Autodesk Inventor part; units mm, degrees
ref_plane "Počáteční rovina" through (0, 0, 0) normal (0, 0, 1) x (1, 0, 0)
ref_plane "Koncová rovina" through (0, 0, 1075) normal (0, 0, 1) x (1, 0, 0)
ref_plane "YZ Plane" through (0, 0, 0) normal (1, 0, 0) x (0, 1, 0)
ref_plane "Počáteční rovina" through (0, 0, 0) normal (0, 0, 1) x (1, 0, 0)
ref_plane "Koncová rovina" through (0, 0, 1075) normal (0, 0, 1) x (1, 0, 0)
sketch "Náčrt1" plane through (0, 0, 0) normal (0, 0, 1) x (1, 0, 0)
  line L0 (-11.5, 17.5) -> (11.5, 17.5)
  line L1 (17.5, 11.5) -> (17.5, -11.5)
  line L2 (11.5, -17.5) -> (-11.5, -17.5)
  line L3 (-17.5, -11.5) -> (-17.5, 11.5)
  arc A0 (-11.5, 17.5) -> (-17.5, 11.5) centre (-11.5, 11.5) ccw
  arc A1 (17.5, 11.5) -> (11.5, 17.5) centre (11.5, 11.5) ccw
  arc A2 (11.5, -17.5) -> (17.5, -11.5) centre (11.5, -11.5) ccw
  arc A3 (-17.5, -11.5) -> (-11.5, -17.5) centre (-11.5, -11.5) ccw
  line L4 (-21.8698, 0) -> (21.8698, 0) construction
  line L5 (0, -21.8698) -> (0, 21.8698) construction
  arc A4 (-11.5, 14.5) -> (-14.5, 11.5) centre (-11.5, 11.5) ccw
  line L6 (-11.5, 14.5) -> (11.5, 14.5)
  arc A5 (14.5, 11.5) -> (11.5, 14.5) centre (11.5, 11.5) ccw
  line L7 (14.5, 11.5) -> (14.5, -11.5)
  arc A6 (11.5, -14.5) -> (14.5, -11.5) centre (11.5, -11.5) ccw
  line L8 (11.5, -14.5) -> (-11.5, -14.5)
  arc A7 (-14.5, -11.5) -> (-11.5, -14.5) centre (-11.5, -11.5) ccw
  line L9 (-14.5, -11.5) -> (-14.5, 11.5)
  point P0 (-17.5, 17.5)
  point P1 (17.5, -17.5)
  point P2 (17.5, 17.5)
  dimension "b" = 35
  dimension "msp_r" = 6
  dimension "d8" = 17.5
  dimension "d9" = 17.5
  dimension "d10" = 3
extrude "Těleso" add sketch "Náčrt1" along normal up to surface (1075 mm away) from surface at 0
sketch "Sketch2" plane through (0, 0, 0) normal (0, 0, 1) x (1, 0, 0)
  line L0 (0, 0) -> (10, 0)
ref_plane "Work Plane3" through (0, 0, 0) normal (0, -1, 0) x (1, 0, 0)
sketch "Sketch3" plane through (0, 0, 0) normal (0, -1, 0) x (1, 0, 0)
  line L0 (-2, 0) -> (12, 0)
  line L1 (-2, 1075) -> (12, 1075)
  dimension "d14" = 1075
sketch "Náčrt4" plane through (11.5, 17.5, 1075) normal (0, 1, 0) x (1, 0, 0)
  line L0 (-23, 1075) -> (-29, 1075)
  line L1 (6, 1075) -> (6, 0)
  line L2 (-29, 1075) -> (6, 1075)
  line L3 (6, 1075) -> (6, 1040.0004)
  line L4 (-29, 1075) -> (6, 1040.0004)
  line L5 (6, 0) -> (6, 35)
  line L6 (-23, 0) -> (-29, 0)
  line L7 (-29, 0) -> (6, 35)
  line L8 (-29, 0) -> (6, 0)
  point P0 (-11.5, 1075)
  point P1 (-26, 0)
  dimension "d15" = 45
  dimension "d16" = 45
extrude "Vysunutí2" cut sketch "Náčrt4" against normal through all
equation "\"msp_r\" = 2 * ParT"
equation "\"d8\" = d9"
equation "\"d9\" = 0.5 * b"
equation "\"d10\" = ParT"
equation "\"G_OFFSET_START\" = 0"
equation "\"G_OFFSET_END\" = 0"
equation "\"d12\" = G_OFFSET_END + B_L"
equation "\"G_L\" = d14"
equation "\"B_L\" = 1075"
properties part number "CSN 426935 - 35x35x3-1075" material "Nerezová ocel"
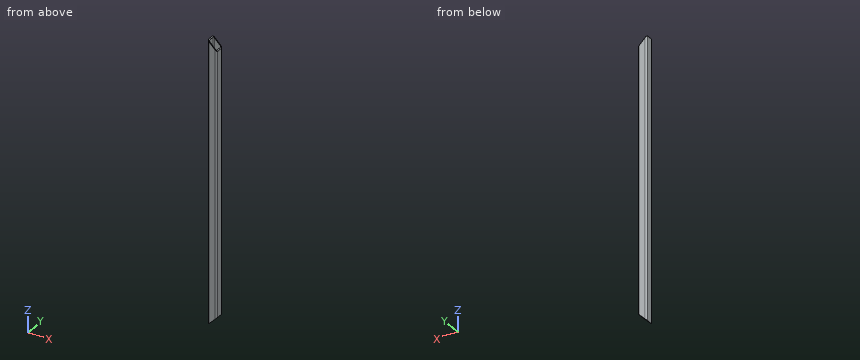
Can you work these out from the model? Positions are in its coordinate system, mm. Coordinates: 2 decimals unless noted, no trailing zeros. Write each loop counter-clockwise with the first axis right and the second up, starting at its lowest first coordinate (ties: lowest second). Pieces come first, ordered by that corner, then holes. Notation, with made-up numbers: M 26.25,84 L 41.25,84 A20 cw 41.25,98 Z; hole C 41,75.25 d6. An arc over 180 degrees is marked long. Write item = value, one per line. Start each with the question number.
Q1. If we section it at B-B, the plane z = 65.5: Write out the boundary of the cut face in (x, y).
Q2. If I drill on L1, parallel to Y at x = 10, z = 568.5; L2, parallel to Y at x = 12.5, z = 903, over which ranges is the centre line in solid material (lowest first)? Write a range as [from, to].
Q3. If we section it at A-A, the plane y = 5: Write out the boundary of the cut face in (x, z), then the cut area to 3 significant figures.
Q4. If we section it at C-C, the plane x = -4.5: Write out the boundary of the cut face in (y, z).
Q5. I'm going to push a flat-ended pin straight in: pin 1 (5 mm diameter, centred on x = -12.5, y = 9.5, fed in from +Z). Where does the tip first touch, or does it pass through?
Check sheet entries:
q1.outline = M -17.5,-11.5 A6 ccw -11.5,-17.5 L 11.5,-17.5 A6 ccw 17.5,-11.5 L 17.5,11.5 A6 ccw 11.5,17.5 L -11.5,17.5 A6 ccw -17.5,11.5 Z; hole M -14.5,-11.5 A3 ccw -11.5,-14.5 L 11.5,-14.5 A3 ccw 14.5,-11.5 L 14.5,11.5 A3 ccw 11.5,14.5 L -11.5,14.5 A3 ccw -14.5,11.5 Z
q2.L1 = [-17.5, -14.5], [14.5, 17.5]
q2.L2 = [-17.42, -14.33], [14.33, 17.42]
q3.outline = M -17.5,0 L -14.5,3 L -14.5,1072 L -17.5,1075 Z; M 14.5,32 L 17.5,35 L 17.5,1040 L 14.5,1043 Z
q3.area = 6,240 mm²
q4.outline = M -17.5,13 L -14.5,13 L -14.5,1062 L -17.5,1062 Z; M 14.5,13 L 17.5,13 L 17.5,1062 L 14.5,1062 Z
q5.pin_1 = 1072.5
